The model under review builds one solid part; all positions refer to its coordinate system, in mm. A direction names the side the tool comes from. Give positions to 0.01 mm unless a question says otherwise; leave off trailing zeros. Order: outer loops, then holes, each group sorted by start corner. A loop starts at its lowest first (then second) coordinate and runs counter-clockwise, first axis right, second up. Notation, with made-up numbers: (35.25, -25) - (74.25, -25) arc R18 cw to (74.25, -3) - close; hole circle Ø1 at (69, 10.25). An arc over 180 degrees is marked (long way). Put each result on its own line as item: value.
```python
from build123d import *

# Parameters (mm, degrees)
SKETCH1_R           = 18.35
BOSS_EXTRUDE1_DEPTH = 21
SHELL1_T            = -1
SKETCH3_R           = 1.5
CUT_EXTRUDE2_DEPTH  = 1
CIRPATTERN1_COUNT   = 6
SKETCH4_R           = 5.9
CUT_EXTRUDE3_DEPTH  = 10
SKETCH5_W           = 11.949895398
SKETCH5_H           = 8
BOSS_EXTRUDE2_DEPTH = 2
SKETCH6_R           = 2
CUT_EXTRUDE4_DEPTH  = 2


with BuildPart() as part:
    # Sketch1 → Boss-Extrude1 (new body)
    with BuildSketch(Plane(origin=(0, 0, 0), x_dir=(0, 0, -1), z_dir=(1, 0, 0))):
        Circle(SKETCH1_R)
    extrude(amount=-BOSS_EXTRUDE1_DEPTH)

    # Shell1
    shell1_openings = [part.faces().sort_by_distance(p)[0] for p in [
        (-21, 0, 0),
    ]]
    offset(amount=SHELL1_T, openings=shell1_openings, kind=Kind.INTERSECTION)

    # Sketch3 → Cut-Extrude2 (cut)
    with BuildSketch(Plane(origin=(0, 0, 0), x_dir=(0, 0, -1), z_dir=(1, 0, 0))):
        with Locations((-7.75, 13.423393759)):
            Circle(SKETCH3_R)
    cut_extrude2 = extrude(amount=-CUT_EXTRUDE2_DEPTH, mode=Mode.SUBTRACT)

    # CirPattern1: Cut-Extrude2 ×6 about axis
    cirpattern1_axis = Axis((0, 0, 0), (1, 0, 0))
    for i in range(1, CIRPATTERN1_COUNT):
        add(cut_extrude2.rotate(cirpattern1_axis, i * 360 / CIRPATTERN1_COUNT), mode=Mode.SUBTRACT)

    # Sketch4 → Cut-Extrude3 (cut)
    with BuildSketch(Plane(origin=(0, 0, 0), x_dir=(0, 0, -1), z_dir=(1, 0, 0))):
        with Locations((0, -7)):
            Circle(SKETCH4_R)
    extrude(amount=-CUT_EXTRUDE3_DEPTH, mode=Mode.SUBTRACT)

    # Sketch5 → Boss-Extrude2 (add)
    with BuildSketch(Plane.ZY.offset(21)):
        with Locations((0, 21.35)):
            Rectangle(SKETCH5_W, SKETCH5_H)
    boss_extrude2 = extrude(amount=-BOSS_EXTRUDE2_DEPTH)

    # Sketch6 → Cut-Extrude4 (cut)
    with BuildSketch(Plane(origin=(-19, 0, 0), x_dir=(0, 0, -1), z_dir=(1, 0, 0))):
        with Locations((0, 21.763901495)):
            Circle(SKETCH6_R)
    cut_extrude4 = extrude(amount=-CUT_EXTRUDE4_DEPTH, mode=Mode.SUBTRACT)

    # Mirror1: Boss-Extrude2, Cut-Extrude4 across plane
    add(boss_extrude2.mirror(Plane.ZX))
    add(cut_extrude4.mirror(Plane.ZX), mode=Mode.SUBTRACT)


solid = part.part
```
(1) For faces 1 (the flat face through (-20, 21, 5.975)), 2 (the flat face through (-20, 21, -5.975)), 3 (the cylindrical face through (-10.86, 17.202, 2.259)), 4 (the flat face through (-20, -21, -5.975)), list the 3-axis set-ups (+Z, -Z, +X, -X, +Y, -Y) from which the entire face can be reached by the end or side of a thin tool; tool diameter is ignored.
The answers:
face 1: +Z, +X, -X, +Y
face 2: -Z, +X, -X, +Y
face 3: -X
face 4: -Z, +X, -X, -Y
(2) Wall thickness on L1, parallel to Y at x = -12.5, z = -0.5; L2, parallel to Y at x = -0.15, z = -7.75; L3, parallel to Y at x = -0.15, z = 0: over which ranges is each line inside the solid? List them lowest first.
The answers:
L1: -18.34 to -17.34, 17.34 to 18.34
L2: -16.63 to -14.92, -11.92 to 11.92, 14.92 to 16.63
L3: -18.35 to -12.9, -1.1 to 18.35
(3) Take a section at D-D, the plane z = 7.75. Write out the cut boundary in (x, y), then the cut area to 3 significant figures.
The answers:
outline: (-21, -16.63) - (0, -16.63) - (0, -14.92) - (-1, -14.92) - (-1, -15.52) - (-21, -15.52) - close; (-21, 15.52) - (-1, 15.52) - (-1, 14.92) - (0, 14.92) - (0, 16.63) - (-21, 16.63) - close; (-1, -11.92) - (0, -11.92) - (0, 11.92) - (-1, 11.92) - close
area: 71.7 mm^2
(4) The part is to be moulded in two halves that separate along Y. For faces 5 (the flat face through (-1, 0, 0)), 6 (the flat face through (-21, -17, -4.2)), 7 (the flat face through (-20, 25.35, 0)), say which applies: pulls with the +Y half, pulls with the -Y half, needs draft (parallel to the pull), parting line crosses it, or undercut.
The answers:
face 5: undercut
face 6: needs draft
face 7: pulls with the +Y half
(5) Clearance check with flat-ended pins moving along their axes: pin 1 Ø3 at (y, z) = (2.5, -13) entering from -X; pin 2 Ø2.5 at (y, z) = (0, 15.5) entering from +X; pin 3 Ø1.6 at (x, y) = (-19.5, 21.5) entering from +Z; pin 4 Ø12 at (x, z) = (-3, -2) entering from +Y. State where each tip first meets the part, or that it passes through.
The answers:
pin 1: x = -1
pin 2: through
pin 3: z = 5.97
pin 4: y = 18.35
(6) Take a section at B-B, the plane z = 0. Write out the cut boundary in (x, y).
The answers:
outline: (-21, -25.35) - (-19, -25.35) - (-19, -23.76) - (-21, -23.76) - close; (-21, -19.76) - (-19, -19.76) - (-19, -18.35) - (0, -18.35) - (0, -12.9) - (-1, -12.9) - (-1, -17.35) - (-21, -17.35) - close; (-21, 17.35) - (-1, 17.35) - (-1, -1.1) - (0, -1.1) - (0, 18.35) - (-19, 18.35) - (-19, 19.76) - (-21, 19.76) - close; (-21, 23.76) - (-19, 23.76) - (-19, 25.35) - (-21, 25.35) - close
(7) Take a section at A-A, the plane y = 0. Write out the cut boundary in (x, z), then the cut area to 3 significant figures.
The answers:
outline: (-21, -18.35) - (0, -18.35) - (0, -17) - (-1, -17) - (-1, -17.35) - (-21, -17.35) - close; (-21, 17.35) - (-1, 17.35) - (-1, 17) - (0, 17) - (0, 18.35) - (-21, 18.35) - close; (-1, -14) - (0, -14) - (0, 14) - (-1, 14) - close
area: 70.7 mm^2
(8) Take a section at C-C, the plane z = 15.5. Write out the cut boundary in (x, y).
The answers:
outline: (-21, -9.82) - (0, -9.82) - (0, -1.5) - (-1, -1.5) - (-1, -7.8) - (-21, -7.8) - close; (-21, 7.8) - (-1, 7.8) - (-1, 1.5) - (0, 1.5) - (0, 9.82) - (-21, 9.82) - close
